CAD build for the part. Positions are in the model's coordinates, mm. Round coordinates to 2 decimals unless told otherwise and drop trailing zeros. Loops run counter-clockwise (first coordinate to the right, second up) from the corner with the lowest first, then second, coordinate; pieces in that order, holes last. Notation, with made-up numbers: (40.5, 48.5) - (61.5, 48.5) arc R21 cw to (61.5, 56.5) - close; hole circle Ø3 at (-5, -14.5). An arc over 180 degrees is marked (long way). Use one line per item in the form item = value.
from build123d import *

# Parameters (mm, degrees)
SKETCH_1_R      = 1.55
SKETCH_1_R_2    = 4.5
SKETCH_1_R_3    = 5
SKETCH_1_W      = 29
SKETCH_1_H      = 8
EXTRUDE_1_DEPTH = 2
FILLET_1_R      = 1


with BuildPart() as part:
    # 草图1 → 凸台-拉伸1 (new body)
    with BuildSketch(Plane.XY):
        Polygon((0, 0), (-80, 0), (-80, 25), (-25, 61), (0, 61), (0, 57.5), (12, 50.57179677), (12, 45), (33.5, 45), (33.5, 29.5), (12, 29.5), (12, 5.595691898), align=None)
        with Locations((-36, 12.5)):
            Circle(SKETCH_1_R, mode=Mode.SUBTRACT)
        with Locations((-56, 12.5)):
            Circle(SKETCH_1_R, mode=Mode.SUBTRACT)
        with Locations((-76, 12.5)):
            Circle(SKETCH_1_R, mode=Mode.SUBTRACT)
        with Locations((-16, 12.5)):
            Circle(SKETCH_1_R, mode=Mode.SUBTRACT)
        with Locations((29.5, 41.5)):
            Circle(SKETCH_1_R, mode=Mode.SUBTRACT)
        with Locations((29.5, 33.5)):
            Circle(SKETCH_1_R, mode=Mode.SUBTRACT)
        with Locations((-5, 33)):
            Circle(SKETCH_1_R, mode=Mode.SUBTRACT)
        with Locations((-20, 33)):
            Circle(SKETCH_1_R, mode=Mode.SUBTRACT)
        with Locations((-5, 45)):
            Circle(SKETCH_1_R, mode=Mode.SUBTRACT)
        with Locations((-20, 45)):
            Circle(SKETCH_1_R, mode=Mode.SUBTRACT)
        with Locations((-5, 57)):
            Circle(SKETCH_1_R, mode=Mode.SUBTRACT)
        with Locations((-20, 57)):
            Circle(SKETCH_1_R, mode=Mode.SUBTRACT)
        with Locations((-26, 8)):
            Circle(SKETCH_1_R_2, mode=Mode.SUBTRACT)
        with Locations((-46, 8)):
            Circle(SKETCH_1_R_2, mode=Mode.SUBTRACT)
        with Locations((-66, 8)):
            Circle(SKETCH_1_R_2, mode=Mode.SUBTRACT)
        with Locations((-2.5, 10)):
            Circle(SKETCH_1_R_3, mode=Mode.SUBTRACT)
        with Locations((-32.5, 32.5)):
            Circle(SKETCH_1_R, mode=Mode.SUBTRACT)
        with Locations(Location((7.5, 32.5, 0), (0, 0, 180))):
            Circle(SKETCH_1_R, mode=Mode.SUBTRACT)
        with Locations((-12.5, 25)):
            Rectangle(SKETCH_1_W, SKETCH_1_H, mode=Mode.SUBTRACT)
        with BuildLine():
            Line((20.5, 34), (12, 34))
            ThreePointArc((12, 34), (8.75, 37.25), (12, 40.5))
            Line((12, 40.5), (20.5, 40.5))
            ThreePointArc((20.5, 40.5), (23.75, 37.25), (20.5, 34))
        make_face(mode=Mode.SUBTRACT)
    extrude(amount=EXTRUDE_1_DEPTH)

    # 圆角1
    fillet_1_edges = [part.edges().sort_by_distance(p)[0] for p in [
        (0, 0, 1),
        (-80, 0, 1),
        (-80, 25, 1),
        (-25, 61, 1),
        (0, 61, 1),
        (0, 57.5, 1),
        (12, 50.57179677, 1),
        (33.5, 45, 1),
        (33.5, 29.5, 1),
        (12, 29.5, 1),
        (12, 5.595691898, 1),
        (-27, 29, 1),
        (-27, 21, 1),
        (2, 21, 1),
        (2, 29, 1),
    ]]
    fillet(fillet_1_edges, radius=FILLET_1_R)


solid = part.part
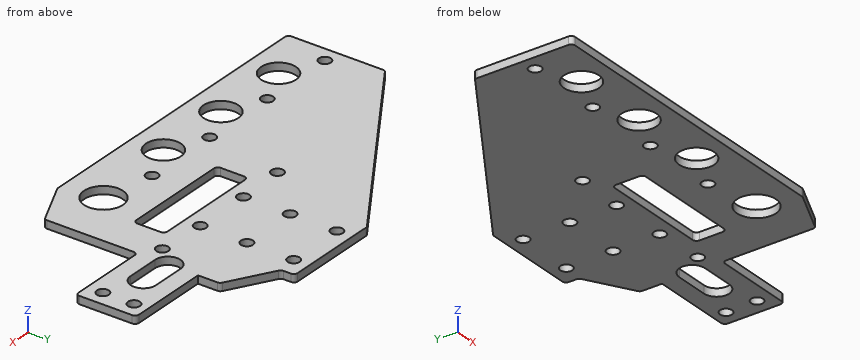
1) Drill centre lines: probe 1 along Y at (x, z) = (-20, 0.55); probe 2 along Y at (x, z) = (-13, 1.05); probe 3 along X at (y, z) = (10.5, 0.15). Where is each one in solid material? Low to high.
Report:
probe_1 = 0 to 21, 29 to 31.45, 34.55 to 43.45, 46.55 to 55.45, 58.55 to 61
probe_2 = 0 to 21, 29 to 61
probe_3 = -80 to -69.74, -62.26 to -49.74, -42.26 to -29.74, -22.26 to -7.47, 2.47 to 12
2) Slice it at A-A (x = -16). Write the cut outline in (y, z).
Report:
outline = (0, 0) - (10.95, 0) - (10.95, 2) - (0, 2) - close; (14.05, 0) - (21, 0) - (21, 2) - (14.05, 2) - close; (29, 0) - (61, 0) - (61, 2) - (29, 2) - close
3) Flat gauge pins, fed straight in: pin 1 (2.5 mm diameter, centred on x = -36, y = 12.5, fed in from -Z); pin 2 (1 mm diameter, centred on y = 14, z = 0.5, fed in from +X). Where does each tip first touch, or does it go through?
Report:
pin_1 = through
pin_2 = 12
4) Slice it at B-B (x = 18.5). Write the cut outline in (y, z).
Report:
outline = (29.5, 0) - (34, 0) - (34, 2) - (29.5, 2) - close; (40.5, 0) - (45, 0) - (45, 2) - (40.5, 2) - close
5) Slice it at D-D (y = 17). Write the cut outline in (x, z), plus the area to 3 significant figures.
Report:
outline = (-80, 0) - (12, 0) - (12, 2) - (-80, 2) - close
area = 184 mm^2
6) Slice it at C-C (z = 1.6). State how many separate pieces and enclosed holes the cut face has, plus the area to 3 significant figures.
Report:
separate_pieces = 1
enclosed_holes = 20
area = 4,140 mm^2
